Build history of the part. All positions in model axes, mm. Face numbers are marked on the shaded views. A direction names the side the tool comes from. Coordinates: 2 decimals unless noted, no trailing zeros. Loops run counter-clockwise (first coordinate to the right, second up) from the corner with the lowest first, then second, coordinate; pieces in that order, holes last.
(1) Slice it at C-C (z = 6.5). Give the cut face in (x, y), and give its area (3 significant figures).
(2) Flat gauge pins, fed straight in: P1, Ø1.5, axis at x = 0, z = 34.5, coming from the +Y side; P2, Ø12, axis at x = 58.5, z = -15, coming from the -Y side; P3, Ø1.5, axis at x = -53.5, z = -28, coming from the +Y side; P4, Ø5.5, axis at x = 50, z = -5.5, coming from the +Y side. Where does each tip first touch, or does it go through?
(3) Slice it at A-A (y = 7). Give the number of separate pieces and of enclosed holes in the cut face, and give its area (3 significant figures).
(4) Slice it at D-D (x = 65). Give the cut face in (y, z).
(5) Two-plate mould, pull along Z, no slides. Class the marked faces 1 and 2: pulls with the +Z half, pulls with the -Z half, needs draft (parallel to the pull), parting line crosses it, or undercut.
(6) Wall check: L1, parallel to X at y = 4.5, z = -19.5; L2, parallel to X at y = 7.5, z = 16.5; L3, parallel to Y at x = -42, z = -3. Give the ranges that are in metal, low to high.
(7) Tool access for the marked faces 3 and 4: list every direction of +Z, -Z, +X, -X, +Y, -Y with a clear straight run to the whole face (end or side of a thin tool).
(8) Slice it at B-B (x = 11). Give the cut face in (y, z), and give its area (3 significant figures).
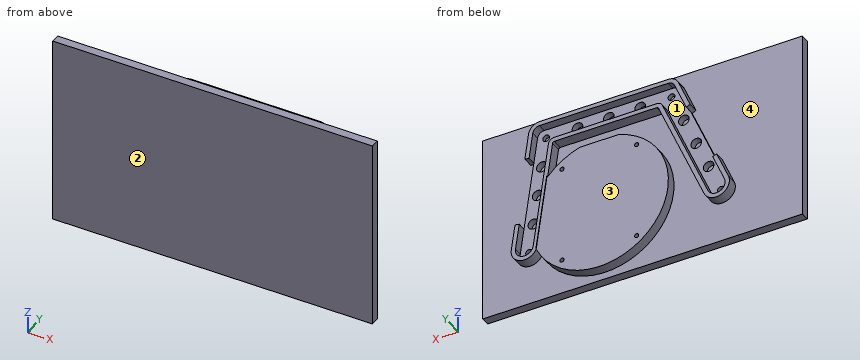
from build123d import *

# Parameters (mm, degrees)
SKETCH1_W           = 150
SKETCH1_H           = 90
BOSS_EXTRUDE1_DEPTH = 4
BOSS_EXTRUDE3_START = 4
BOSS_EXTRUDE3_DEPTH = 1
SKETCH3_R           = 1.6
CUT_EXTRUDE3_DEPTH  = 2
SKETCH5_R           = 2.5
CUT_EXTRUDE4_DEPTH  = 3.25
BOSS_EXTRUDE2_DEPTH = 5
CUT_EXTRUDE5_REACH  = 89.926
SKETCH10_R          = 1
BOSS_EXTRUDE4_DEPTH = 4.7244
CUT_EXTRUDE6_DEPTH  = 0.2756


# Read off the part's stored shape, not the designer's step: Boss-Extrude3
with BuildPart() as part:
    # Sketch1 → Boss-Extrude1 (new body)
    with BuildSketch(Plane(origin=(0, 0, 0), x_dir=(1, 0, 0), z_dir=(0, 1, 0))):
        Rectangle(SKETCH1_W, SKETCH1_H)
    extrude(amount=BOSS_EXTRUDE1_DEPTH)

    # Boss-Extrude3 outline → Boss-Extrude3 (add)
    with BuildSketch(Plane(origin=(0, 0, 0), x_dir=(1, 0, 0), z_dir=(0, 1, 0)).offset(BOSS_EXTRUDE3_START)):
        with BuildLine():
            ThreePointArc((-33.446001745, 21.59344723), (-38.948165427, 23.830899981), (-41.185618178, 18.328736299))
            Line((-41.185618178, 18.328736299), (-17.72774219, -37.282607638))
            ThreePointArc((-17.72774219, -37.282607638), (-16.548520363, -38.70535138), (-14.779316882, -39.238908236))
            Line((-14.779316882, -39.238908236), (45.549258637, -39.238908236))
            ThreePointArc((45.549258637, -39.238908236), (47.642826881, -38.459026417), (48.715935243, -36.499515742))
            Line((48.715935243, -36.499515742), (56.840453083, 19.356544412))
            ThreePointArc((56.840453083, 19.356544412), (53.28873739, 24.117354809), (48.527926993, 20.565639116))
            Line((48.527926993, 20.565639116), (41.399551878, -28.441939804))
            ThreePointArc((41.399551878, -28.441939804), (40.460582061, -30.156511644), (38.628709848, -30.838908236))
            Line((38.628709848, -30.838908236), (-9.471261516, -30.838908236))
            ThreePointArc((-9.471261516, -30.838908236), (-11.019314561, -30.372045987), (-12.05113366, -29.127145213))
            Line((-12.05113366, -29.127145213), (-33.446001745, 21.59344723))
        make_face()
    extrude(amount=BOSS_EXTRUDE3_DEPTH)

    # Sketch3 → Cut-Extrude3 (cut)
    with BuildSketch(Plane(origin=(0, 5, 0), x_dir=(1, 0, 0), z_dir=(0, 1, 0))):
        with Locations(Location((-37.315809962, 19.961091764, 0), (0, 0, 270))):
            Circle(SKETCH3_R)
        with Locations(Location((-14.115809962, -35.038908236, 0), (0, 0, 270))):
            Circle(SKETCH3_R)
        with Locations(Location((44.684190038, -35.038908236, 0), (0, 0, 270))):
            Circle(SKETCH3_R)
        with Locations(Location((52.684190038, 19.961091764, 0), (0, 0, 270))):
            Circle(SKETCH3_R)
    extrude(amount=-CUT_EXTRUDE3_DEPTH, mode=Mode.SUBTRACT)

    # Sketch5 → Cut-Extrude4 (cut)
    with BuildSketch(Plane(origin=(0, 5, 0), x_dir=(1, 0, 0), z_dir=(0, 1, 0))):
        with Locations(Location((-31.515809962, 6.211091764, 0), (0, 0, 270))):
            Circle(SKETCH5_R)
        with Locations(Location((15.284190038, -35.038908236, 0), (0, 0, 270))):
            Circle(SKETCH5_R)
        with Locations(Location((46.684190038, -21.288908236, 0), (0, 0, 270))):
            Circle(SKETCH5_R)
        with Locations(Location((-19.915809962, -21.288908236, 0), (0, 0, 270))):
            Circle(SKETCH5_R)
        with Locations(Location((50.684190038, 6.211091764, 0), (0, 0, 270))):
            Circle(SKETCH5_R)
        with Locations(Location((-25.715809962, -7.538908236, 0), (0, 0, 270))):
            Circle(SKETCH5_R)
        with Locations(Location((0.584190038, -35.038908236, 0), (0, 0, 270))):
            Circle(SKETCH5_R)
        with Locations(Location((29.984190038, -35.038908236, 0), (0, 0, 270))):
            Circle(SKETCH5_R)
        with Locations(Location((48.684190038, -7.538908236, 0), (0, 0, 270))):
            Circle(SKETCH5_R)
    extrude(amount=-CUT_EXTRUDE4_DEPTH, mode=Mode.SUBTRACT)

    # Sketch6 → Boss-Extrude2 (add)
    with BuildSketch(Plane(origin=(0, 4, 0), x_dir=(1, 0, 0), z_dir=(0, 1, 0))):
        with BuildLine():
            Line((46.548754115, 20.853518808), (39.420378999, -28.154060112))
            ThreePointArc((39.420378999, -28.154060112), (39.152101909, -28.643937781), (38.628709848, -28.838908236))
            Line((38.628709848, -28.838908236), (-9.471261516, -28.838908236))
            ThreePointArc((-9.471261516, -28.838908236), (-9.913562386, -28.705519022), (-10.208367842, -28.349833086))
            Line((-10.208367842, -28.349833086), (-31.603235928, 22.370759357))
            ThreePointArc((-31.603235928, 22.370759357), (-39.725477554, 25.673665798), (-43.028383996, 17.551424172))
            Line((-43.028383996, 17.551424172), (-19.570508008, -38.059919765))
            ThreePointArc((-19.570508008, -38.059919765), (-17.654272538, -40.371878346), (-14.779316882, -41.238908236))
            Line((-14.779316882, -41.238908236), (45.549258637, -41.238908236))
            ThreePointArc((45.549258637, -41.238908236), (48.951307033, -39.97160028), (50.695108121, -36.787395433))
            Line((50.695108121, -36.787395433), (58.819625962, 19.068664721))
            ThreePointArc((58.819625962, 19.068664721), (53.576617082, 26.096527688), (46.548754115, 20.853518808))
        make_face()
        with BuildLine():
            Line((-9.471261516, -30.838908236), (38.628709848, -30.838908236))
            ThreePointArc((38.628709848, -30.838908236), (40.460582061, -30.156511644), (41.399551878, -28.441939804))
            Line((41.399551878, -28.441939804), (48.527926993, 20.565639116))
            ThreePointArc((48.527926993, 20.565639116), (53.28873739, 24.117354809), (56.840453083, 19.356544412))
            Line((56.840453083, 19.356544412), (48.715935243, -36.499515742))
            ThreePointArc((48.715935243, -36.499515742), (47.642826881, -38.459026417), (45.549258637, -39.238908236))
            Line((45.549258637, -39.238908236), (-14.779316882, -39.238908236))
            ThreePointArc((-14.779316882, -39.238908236), (-16.548520363, -38.70535138), (-17.72774219, -37.282607638))
            Line((-17.72774219, -37.282607638), (-41.185618178, 18.328736299))
            ThreePointArc((-41.185618178, 18.328736299), (-38.948165427, 23.830899981), (-33.446001745, 21.59344723))
            Line((-33.446001745, 21.59344723), (-12.05113366, -29.127145213))
            ThreePointArc((-12.05113366, -29.127145213), (-11.019314561, -30.372045987), (-9.471261516, -30.838908236))
        make_face(mode=Mode.SUBTRACT)
    extrude(amount=BOSS_EXTRUDE2_DEPTH)

    # Cut-Extrude5: up to this face of the body (flat: up to its plane)
    cut_extrude5_end = Plane(part.part.faces().sort_by_distance((-2.356631327, 4, -3.006871304))[0])
    # Sketch9 → Cut-Extrude5 (cut, up to the picked face)
    with BuildSketch(Plane(origin=(0, 9, 0), x_dir=(1, 0, 0), z_dir=(0, 1, 0)), mode=Mode.PRIVATE) as cut_extrude5_sk1:
        Polygon((-23.238183171, -24.219062209), (-35.675177197, 5.26519087), (-37.517943015, 4.487878743), (-25.080948989, -24.996374336), align=None)
    cut_extrude5_tool1 = split(extrude(cut_extrude5_sk1.sketch, amount=-CUT_EXTRUDE5_REACH, mode=Mode.PRIVATE), bisect_by=cut_extrude5_end, keep=Keep.BOTH, mode=Mode.PRIVATE)
    # Sketch9 → Cut-Extrude5 (cut, up to the picked face)
    with BuildSketch(Plane(origin=(0, 9, 0), x_dir=(1, 0, 0), z_dir=(0, 1, 0)), mode=Mode.PRIVATE) as cut_extrude5_sk2:
        Polygon((55.081231695, 7.261897364), (50.475156632, -24.404868693), (52.45432951, -24.692748385), (57.060404573, 6.974017672), align=None)
    cut_extrude5_tool2 = split(extrude(cut_extrude5_sk2.sketch, amount=-CUT_EXTRUDE5_REACH, mode=Mode.PRIVATE), bisect_by=cut_extrude5_end, keep=Keep.BOTH, mode=Mode.PRIVATE)
    add(cut_extrude5_tool1.solids().sort_by(Axis((-30.378063, 9, 9.865592), (0, -1, 0)))[0], mode=Mode.SUBTRACT)
    add(cut_extrude5_tool2.solids().sort_by(Axis((53.767781, 9, 8.715426), (0, -1, 0)))[0], mode=Mode.SUBTRACT)

    # Sketch10 → Boss-Extrude4 (add)
    with BuildSketch(Plane(origin=(0, 4, 0), x_dir=(1, 0, 0), z_dir=(0, 1, 0))):
        with BuildLine():
            Line((8.603375751, -21.785908236), (26.725004326, -21.785908236))
            ThreePointArc((26.725004326, -21.785908236), (34.872763222, -18.130879321), (41.713269692, -12.390436602))
            Line((41.713269692, -12.390436602), (46.548754115, 20.853518808))
            ThreePointArc((46.548754115, 20.853518808), (46.771885392, 21.8278145), (47.148675016, 22.753594842))
            ThreePointArc((47.148675016, 22.753594842), (-6.835267399, 30.523629914), (8.603375751, -21.785908236))
        make_face()
        with Locations(Location((0.164190038, 32.321352082, 0), (0, 0, 270))):
            Circle(SKETCH10_R, mode=Mode.SUBTRACT)
        with Locations(Location((0.164190038, -13.678647918, 0), (0, 0, 270))):
            Circle(SKETCH10_R, mode=Mode.SUBTRACT)
        with Locations(Location((35.164190038, -13.678647918, 0), (0, 0, 270))):
            Circle(SKETCH10_R, mode=Mode.SUBTRACT)
        with Locations(Location((35.164190038, 32.321352082, 0), (0, 0, 270))):
            Circle(SKETCH10_R, mode=Mode.SUBTRACT)
    extrude(amount=BOSS_EXTRUDE4_DEPTH)

    # Sketch11 → Cut-Extrude6 (cut)
    with BuildSketch(Plane(origin=(0, 9, 0), x_dir=(1, 0, 0), z_dir=(0, 1, 0))):
        Polygon((41.713269692, -12.390436602), (46.831832261, 22.799681061), (47.32662548, 22.727711139), (42.208062911, -12.462406525), align=None)
    extrude(amount=-CUT_EXTRUDE6_DEPTH, mode=Mode.SUBTRACT)


solid = part.part
Response values:
1. outline: (-75, 0) - (75, 0) - (75, 4) - (53.08, 4) - (53.08, 5) - (50.96, 5) - (50.96, 1.75) - (46.41, 1.75) - (46.41, 5) - (44.59, 5) - (44.59, 9) - (43.08, 9) - (43.08, 8.72) - (-10.61, 8.72) - (-10.61, 4) - (-19.43, 4) - (-19.43, 9) - (-21.6, 9) - (-21.6, 5) - (-23.44, 5) - (-23.44, 1.75) - (-27.99, 1.75) - (-27.99, 5) - (-30.71, 5) - (-30.71, 4) - (-75, 4) - close
1. area: 860 mm2
2. P1: stops at y = 1.75
2. P2: stops at y = 0
2. P3: stops at y = 4
2. P4: stops at y = 5
3. separate pieces: 2
3. enclosed holes: 4
3. area: 3,760 mm2
4. outline: (0, -45) - (4, -45) - (4, 45) - (0, 45) - close
5. face 1: undercut
5. face 2: needs draft
6. L1: x = -43.5 to -38.85, -35.78 to -30.39, -13.1 to 51.15, 54.22 to 58.87
6. L2: x = -17.38 to -15.21, -1.91 to 37.24, 41.12 to 43.14
6. L3: y = 0 to 4
7. face 3: -Z, +Y
7. face 4: +Y
8. outline: (0, -45) - (4, -45) - (4, -41.03) - (8.72, -41.03) - (8.72, 21.79) - (4, 21.79) - (4, 28.84) - (9, 28.84) - (9, 30.84) - (5, 30.84) - (5, 39.24) - (9, 39.24) - (9, 41.24) - (4, 41.24) - (4, 45) - (0, 45) - close
8. area: 685 mm2
